Check sheet for the modelled part. Datum: model origin and axes. Units: mm. A direction names the side the tool comes from. Give positions to 0.01 mm unless a question says otherwise; leave off trailing zeros. Write each loop counter-clockwise with the first axis right and the second up, starting at its lowest first coordinate (ties: lowest second). Pieces come first, ordered by that corner, then holes. Notation, with made-up numbers: M 86,36 L 118,36 A23 cw 118,61 Z; hole C 25.25,-22.5 d11. An arc over 180 degrees is marked long. Write each question's results on one line, items separated by ' | '. Start each with the question number.
from build123d import *

# Parameters (mm, degrees)
F0_W     = 85
F0_H     = 85
F1_DEPTH = 85
F2_T     = -0.6
F3_R     = 24.5
F4_DEPTH = 25


with BuildPart() as f1:
    # F0 (on Top) → F1 (new body)
    with BuildSketch(Plane.XY):
        Rectangle(F0_W, F0_H)
    extrude(amount=F1_DEPTH)

    # F2
    f2_openings = [f1.faces().sort_by_distance(p)[0] for p in [
        (0, 0, 85),
    ]]
    offset(amount=F2_T, openings=f2_openings)

    # F3 (on Top) → F4 (cut)
    with BuildSketch(Plane.XY):
        Circle(F3_R)
    extrude(amount=F4_DEPTH, mode=Mode.SUBTRACT)


solid = f1.part
Q1. Release check for a two-part mould opening along Y. For faces 1 (the face through (-1, 42.5, 42)), 2 (the face through (-19, -18, 0)), 3 (the face through (-1, 41.9, 42)) record: pulls with the +Y half, pulls with the -Y half, needs draft (parallel to the pull), parting line crosses it, or undercut.
Q2. Tool access check on faces 4 (the face through (41.9, -1, 42)), 5 (the face through (13.17, 20.66, 0.3)). Record the directions out of +Z, -Z, +X, -X, +Y, -Y that give a thin tool (end or side, any length) a straight path to the whole face; none if there is none.
Q3. Section check D-D on y = 30. Record the boundary of the cut face in (x, z).
Q4. Section check A-A on x = 0. Record the boundary of the cut face in (y, z).
Q5. Scan lines: L1, parallel to X at y = -2.5, z = 32; L2, parallel to Y at x = 0, z = 0.4. Record each from-to range of solid material in increasing order.
Q6. Depth check by flat-ended pin: pin 1 Ø5 at (x, y) = (23, -6) entering from +Z. Enter the tip coordinate at first touch or a pass-through.
Q7. Section check C-C on z = 65. Record the boundary of the cut face in (x, y), plus the area to 3 significant figures.
Check result:
1) face 1: pulls with the +Y half | face 2: needs draft | face 3: undercut
2) face 4: +Z | face 5: +Z, -Z
3) outline: M -42.5,0 L 42.5,0 L 42.5,85 L 41.9,85 L 41.9,0.6 L -41.9,0.6 L -41.9,85 L -42.5,85 Z
4) outline: M -42.5,0 L -24.5,0 L -24.5,0.6 L -41.9,0.6 L -41.9,85 L -42.5,85 Z; M 24.5,0 L 42.5,0 L 42.5,85 L 41.9,85 L 41.9,0.6 L 24.5,0.6 Z
5) L1: -42.5 to -41.9, 41.9 to 42.5 | L2: -42.5 to -24.5, 24.5 to 42.5
6) pin 1: z = 0.6
7) outline: M -42.5,-42.5 L 42.5,-42.5 L 42.5,42.5 L -42.5,42.5 Z; hole M -41.9,-41.9 L 41.9,-41.9 L 41.9,41.9 L -41.9,41.9 Z | area: 203 mm^2
